Read the model definition and answer for the solid it produces. Units are mm, in the model's axes. A direction names the side the tool comes from. Round coordinates to 2 decimals unless told otherwise and drop trailing zeros. Loops run counter-clockwise (first coordinate to the right, second up) from the corner with the lowest first, then second, coordinate; pieces in that order, holes last. Notation, with made-up numbers: (36.5, 24.5) - (55.5, 24.5) arc R28 ccw to (55.5, 45.5) - close; hole circle Ø3 at (64.25, 57). An arc over 180 degrees is marked (long way). Use CSV: the item, a comma, the result in double quotes. Start each with the question number.
1. Determine the mould class of faces 1 (the flat face through (12, 0, 0)), 2 (the cylindrical face through (49.223, 0.231, -8.592)), 3 (the flat face through (-9.525, 0, -21)) for opening direction X: +X half, -X half, draft (parallel to the pull), parting line (faces both ways), or undercut.
2. Consider line 1 along Z through (x, y) = (2, -14.5); line 2 along X through (y, z) = (-10.5, -16) (3 decimals); line 3 along Z through (x, y) = (47, 1). Determine where each line is inside the solid, lowest interval first.
3. A tool of negligible diameter and unlimited length cuts with its end or side. For faces 4 (the flat face through (-9.525, 0, 1)), 5 (the flat face through (12, 0, -19.304)), from which of +Z, -Z, +X, -X, +Y, -Y can it reach the whole face along a straight path? Write none if from no direction.
4. Find section A-A (x = 17). Give the vertices of the cut face in (y, z), and give its area (3 significant figures).
5. Find section C-C (x = 44.45). Give the vertices of the cut face in (y, z).
6. Given pin 1 Ø12 at (y, z) = (2, -10) entering from -X (3 decimals); pin 2 Ø9 at (x, z) = (44.45, -9.652) entering from -Y, each flat-ended and moving along its own axis, determine where each tip first touches the part or whether it passes through.
7. Find section D-D (z = -3.5). Give the vertices of the cut face in (x, y) (3 decimals).
Autodesk Inventor part; units mm, degrees
ref_plane "YZ Plane" through (0, 0, 0) normal (1, 0, 0) x (0, 1, 0)
ref_plane "XZ Plane" through (0, 0, 0) normal (0, 1, 0) x (-1, 0, 0)
ref_plane "XY Plane" through (0, 0, 0) normal (0, 0, 1) x (1, 0, 0)
ref_plane "Work Plane1" through (0, 0, 0) normal (0, 0, 1) x (1, 0, 0)
sketch "Sketch1" plane through (0, 0, 0) normal (0, 0, 1) x (1, 0, 0)
  line L0 (3, 16.51) -> (-3, 16.51) construction
  line L1 (-3, -16.51) -> (3, -16.51) construction
  line L2 (-9.525, -16.51) -> (-9.525, 173.99) construction
  line L3 (9.525, -16.51) -> (9.525, 173.99) construction
  line L4 (-9.525, -16.51) -> (53.975, -16.51)
  line L5 (53.975, -16.51) -> (53.975, 16.51)
  line L6 (53.975, 16.51) -> (-9.525, 16.51)
  line L7 (-9.525, 16.51) -> (-9.525, -16.51)
  point P0 (0, 0)
  dimension "d0" = 63.5
extrude "Extrusion1" add sketch "Sketch1" along normal blind 2.54
ref_plane "Work Plane2" through (0, 0, -19.304) normal (0, 0, -1) x (1, 0, 0)
sketch "Sketch2" plane through (0, 0, -19.304) normal (0, 0, -1) x (1, 0, 0)
  line L0 (-9.525, 16.51) -> (53.975, 16.51)
  line L1 (53.975, -16.51) -> (-9.525, -16.51)
  line L2 (-9.525, 16.51) -> (53.975, 16.51)
  line L3 (53.975, 16.51) -> (53.975, -16.51)
  line L4 (53.975, -16.51) -> (-9.525, -16.51)
  line L5 (-9.525, -16.51) -> (-9.525, 16.51)
  point P0 (0, 0)
  dimension "d3" = 63.5
extrude "Extrusion2" add sketch "Sketch2" along normal blind 2.54
sketch "Sketch3" plane through (-9.525, -16.51, 0) normal (0, -1, 0) x (1, 0, 0)
  line L0 (63.5, 0) -> (0, 0)
  line L1 (0, -19.304) -> (63.5, -19.304)
  line L2 (63.5, 0) -> (44.45, 0)
  line L3 (44.45, 0) -> (44.45, -19.304)
  line L4 (44.45, -19.304) -> (63.5, -19.304)
  line L5 (63.5, -19.304) -> (63.5, 0)
  point P0 (9.525, 0)
  dimension "d6" = 19.05
extrude "Extrusion3" add sketch "Sketch3" against normal blind 33.02
sketch "Sketch4" plane through (-9.525, -16.51, 2.54) normal (0, -1, 0) x (1, 0, 0)
  line L0 (44.45, -21.844) -> (44.45, -2.54) construction
  line L1 (44.45, -12.192) -> (63.5, -12.192) construction
  point P0 (9.525, -2.54)
  point P1 (53.975, -12.192)
hole "Hole1" at (44.45, -16.51, -9.652) direction (0, 1, 0) diameter 9.779 end through all
properties part number "XRailVerticalExtension"
Filled sheet:
1,face 1,"draft"
1,face 2,"undercut"
1,face 3,"-X half"
2,line 1,"z = -21.84 to -19.3, 0 to 2.54"
2,line 2,"x = 34.925 to 53.975"
2,line 3,"z = -21.84 to -13.82, -5.48 to 2.54"
3,face 4,"+Z, -Z, -X, +Y, -Y"
3,face 5,"-X, +Y, -Y"
4,outline,"(-16.51, -21.84) - (16.51, -21.84) - (16.51, -19.3) - (-16.51, -19.3) - close; (-16.51, 0) - (16.51, 0) - (16.51, 2.54) - (-16.51, 2.54) - close"
4,area,"168 mm²"
5,outline,"(-16.51, -21.84) - (16.51, -21.84) - (16.51, -14.54) - (-16.51, -14.54) - close; (-16.51, -4.76) - (16.51, -4.76) - (16.51, 2.54) - (-16.51, 2.54) - close"
6,pin 1,"stops at x = 34.925"
6,pin 2,"passes through"
7,outline,"(34.925, -16.51) - (53.975, -16.51) - (53.975, 16.51) - (34.925, 16.51) - close"
